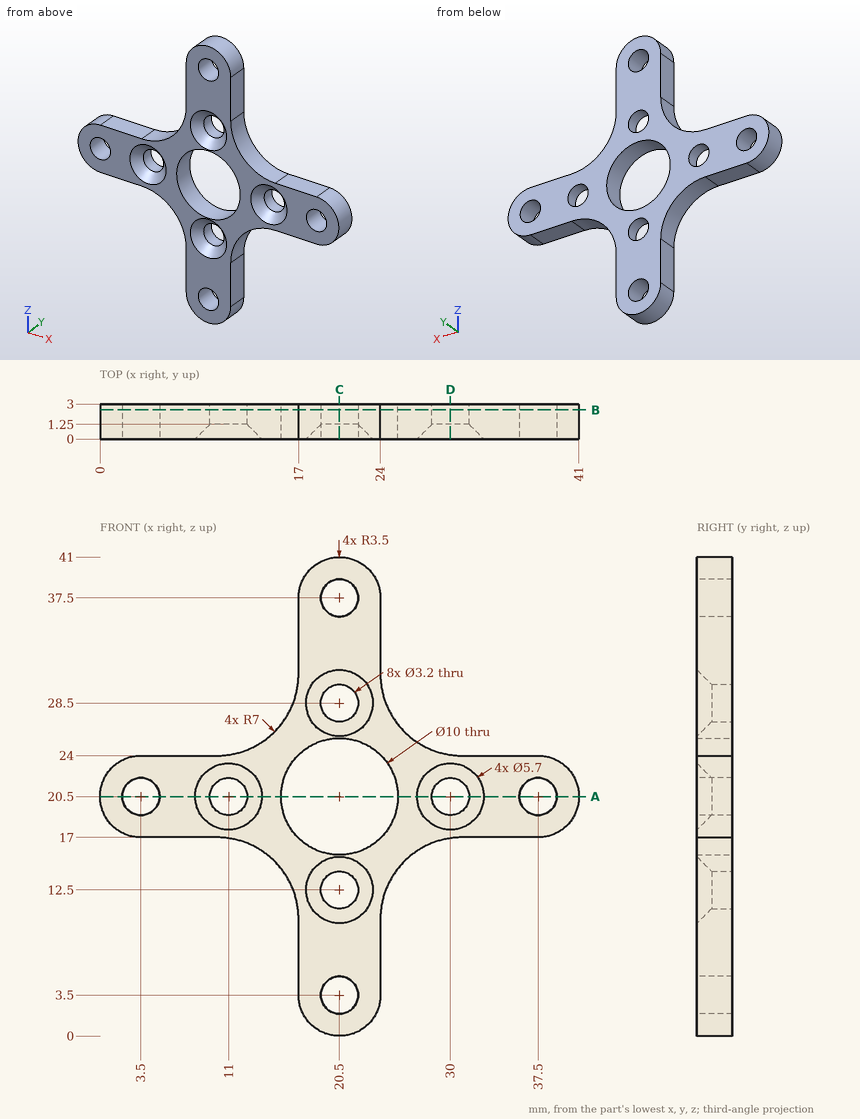
Answer from the drawing. Dimensions are ordinates in mm from the lowest x, y and z of the part. Give positions to 0.01 mm unless a question says otherwise; leave off trailing zeros. Order: outer loops, then holes, each group sorted by start corner. A loop starts at its lowest first (then second) coordinate and runs counter-clockwise, first axis right, second up. Notation, with made-up numbers: (41.5, 73.5) -> (86.5, 73.5) arc R17 ccw to (86.5, 92.5) -> close; hole circle Ø10 at (73.5, 54). An arc over 180 degrees is marked (long way). One line per item, written item: value.
Item 1: Find section B-B, the plane y = 2.5. State how many separate pieces and enclosed holes the cut face has, plus the area to 3 significant figures.
Answer sheet:
separate pieces: 1
enclosed holes: 9
area: 403 mm²
Item 2: Flat-ended cylindrical pins translate along their axes: P1, Ø5, axis at x = 30, z = 20.5, coming from the -Y side; P2, Ø1.5, axis at y = 1, z = 33, coming from the +X side; P3, Ø3, axis at x = 18, z = 15, coming from the -Y side; P4, Ø1.5, axis at x = 34, y = 1.5, coming from the +Z side. Find the tip coordinate at first contact, or state that the pin passes through.
Answer sheet:
P1: y = 0.35
P2: x = 24
P3: y = 0
P4: z = 24
Item 3: Find section A-A, the plane z = 20.5. Give the vertices of the cut face in (x, y), plus the area to 3 significant figures.
Answer sheet:
outline: (0, 0) -> (1.9, 0) -> (1.9, 3) -> (0, 3) -> close; (5.1, 0) -> (8.15, 0) -> (9.4, 1.25) -> (9.4, 3) -> (5.1, 3) -> close; (12.6, 1.25) -> (13.85, 0) -> (15.5, 0) -> (15.5, 3) -> (12.6, 3) -> close; (25.5, 0) -> (27.15, 0) -> (28.4, 1.25) -> (28.4, 3) -> (25.5, 3) -> close; (31.6, 1.25) -> (32.85, 0) -> (35.9, 0) -> (35.9, 3) -> (31.6, 3) -> close; (39.1, 0) -> (41, 0) -> (41, 3) -> (39.1, 3) -> close
area: 51.5 mm²
Item 4: Straight lines are drawn through the part: probe 1 along X at (y, z) = (2.2, 20.5); probe 2 along Z at (x, y) = (37.5, 0.8); probe 3 along X at (y, z) = (0.7, 35). For each, find the intervals that lie inside material, in ascending order.
Answer sheet:
probe 1: 0 to 1.9, 5.1 to 9.4, 12.6 to 15.5, 25.5 to 28.4, 31.6 to 35.9, 39.1 to 41
probe 2: 17 to 18.9, 22.1 to 24
probe 3: 17 to 24
Item 5: Find section C-C, the plane x = 20.5. Give the vertices of the cut face in (y, z).
Answer sheet:
outline: (0, 0) -> (3, 0) -> (3, 1.9) -> (0, 1.9) -> close; (0, 5.1) -> (3, 5.1) -> (3, 10.9) -> (1.25, 10.9) -> (0, 9.65) -> close; (0, 15.35) -> (1.25, 14.1) -> (3, 14.1) -> (3, 15.5) -> (0, 15.5) -> close; (0, 25.5) -> (3, 25.5) -> (3, 26.9) -> (1.25, 26.9) -> (0, 25.65) -> close; (0, 31.35) -> (1.25, 30.1) -> (3, 30.1) -> (3, 35.9) -> (0, 35.9) -> close; (0, 39.1) -> (3, 39.1) -> (3, 41) -> (0, 41) -> close
Item 6: Find section D-D, the plane x = 30. Give the vertices of the cut face in (y, z), plus the area to 3 significant figures.
Answer sheet:
outline: (0, 16.93) -> (3, 16.93) -> (3, 18.9) -> (1.25, 18.9) -> (0, 17.65) -> close; (0, 23.35) -> (1.25, 22.1) -> (3, 22.1) -> (3, 24.07) -> (0, 24.07) -> close
area: 10.3 mm²
